The model under review builds one solid part; all positions refer to its coordinate system, in mm. Face numbers are marked on the shaded views. Coordinates: 2 decimals unless noted, no trailing zeros. Loops run counter-clockwise (first coordinate to the right, second up) from the corner with the lowest first, then second, coordinate; pieces in that order, holes last. Notation, with made-up numbers: M -32.75,39.25 L -19.75,39.25 A12 cw -19.75,43.25 Z; hole C -24.5,31.25 d10. An arc over 180 degrees is marked long. Return JSON: item names as keys, results as strings.
Autodesk Inventor part; units mm, degrees
ref_plane "YZ Plane" through (0, 0, 0) normal (1, 0, 0) x (0, 1, 0)
ref_plane "XZ Plane" through (0, 0, 0) normal (0, 1, 0) x (-1, 0, 0)
ref_plane "XY Plane" through (0, 0, 0) normal (0, 0, 1) x (1, 0, 0)
sketch "Sketch1" plane through (0, 0, 0) normal (0, 1, 0) x (-1, 0, 0)
  line L0 (0, 0) -> (0, -55.5) construction
  circle A0 centre (0, -55.5) radius 8
  line L1 (0, 0) -> (10, 0) construction
  line L2 (0, 0) -> (-10, 0) construction
  line L3 (10, -55.5) -> (10, 0)
  line L4 (-10, -55.5) -> (-10, 0)
  line L5 (0, 0) -> (0, -12.5) construction
  line L6 (0, -12.5) -> (0, -37.5) construction
  line L7 (0, -65.5) -> (0, -69.5) construction
  line L8 (0, -69.5) -> (3.25, -69.5)
  line L9 (4, -68.75) -> (4, -67.5)
  line L10 (0, -69.5) -> (-3.25, -69.5)
  line L11 (-4, -68.75) -> (-4, -67.5)
  arc A1 (-10, -55.5) -> (-6, -63.5) centre (0, -55.5) ccw
  arc A2 (6, -63.5) -> (10, -55.5) centre (0, -55.5) ccw
  arc A3 (6, -63.5) -> (4, -67.5) centre (9, -67.5) ccw
  arc A4 (-4, -67.5) -> (-6, -63.5) centre (-9, -67.5) ccw
  arc A5 (-4, -68.75) -> (-3.25, -69.5) centre (-3.25, -68.75) ccw
  arc A6 (3.25, -69.5) -> (4, -68.75) centre (3.25, -68.75) ccw
  line L12 (0, 0) -> (0, 55.5) construction
  circle A7 centre (0, 55.5) radius 8
  line L13 (10, 55.5) -> (10, 0)
  line L14 (-10, 55.5) -> (-10, 0)
  line L15 (0, 0) -> (0, 12.5) construction
  line L16 (0, 12.5) -> (0, 37.5) construction
  line L17 (0, 65.5) -> (0, 69.5) construction
  line L18 (0, 69.5) -> (3.25, 69.5)
  line L19 (4, 68.75) -> (4, 67.5)
  line L20 (0, 69.5) -> (-3.25, 69.5)
  line L21 (-4, 68.75) -> (-4, 67.5)
  arc A8 (-6, 63.5) -> (-10, 55.5) centre (0, 55.5) ccw
  arc A9 (10, 55.5) -> (6, 63.5) centre (0, 55.5) ccw
  arc A10 (4, 67.5) -> (6, 63.5) centre (9, 67.5) ccw
  arc A11 (-6, 63.5) -> (-4, 67.5) centre (-9, 67.5) ccw
  arc A12 (-3.25, 69.5) -> (-4, 68.75) centre (-3.25, 68.75) ccw
  arc A13 (4, 68.75) -> (3.25, 69.5) centre (3.25, 68.75) ccw
  point P0 (4, -69.5)
  point P1 (4, -64.6652)
  point P2 (-4, -69.5)
  point P3 (-4, -64.6652)
  point P4 (4, 69.5)
  point P5 (4, 64.6652)
  point P6 (-4, 69.5)
  point P7 (-4, 64.6652)
  dimension "d0" = 55.5
  dimension "d1" = 16
  dimension "d3" = 10
  dimension "d4" = 10
  dimension "d6" = 12.5
  dimension "d7" = 25
  dimension "d10" = 4
  dimension "d11" = 4
  dimension "d12" = 4
  dimension "d13" = 5
  dimension "d14" = 0.75
extrude "Extrusion1" add sketch "Sketch1" along normal blind 25
sketch "Sketch2" plane through (0, 0, 0) normal (0, 0, 1) x (1, 0, 0)
  line L0 (-10, 25) -> (10, 18.5016)
  line L1 (10, 0) -> (10, 25)
  line L2 (-10, 25) -> (11.0292, 25) construction
  line L3 (10, 18.5016) -> (10, 25)
  line L4 (10, 25) -> (-10, 25)
  point P0 (0, 0)
  dimension "d17" = 18
extrude "Extrusion2" cut sketch "Sketch2" along normal through all both and the other way through all
sketch "Sketch3" plane through (10, 18.5016, 55.5) normal (0.309, 0.9511, 0) x (0.9511, -0.309, 0)
  ellipse E0 centre (-10.5146, 0) end of major axis (-2.1029, 0) minor radius 8
  ellipse E1 centre (-10.5146, 111) end of major axis (-2.1029, 111) minor radius 8
  line L0 (-10.5146, 0) -> (-10.5146, 111) construction
  line L1 (-10.5146, 55.5) -> (-10.5146, 43)
  line L2 (-10.5146, 43) -> (-10.5146, 18)
  line L3 (-10.5146, 55.5) -> (-10.5146, 68)
  line L4 (-10.5146, 68) -> (-10.5146, 93)
  circle A0 centre (-10.5146, 18) radius 2
  circle A1 centre (-10.5146, 43) radius 2
  circle A2 centre (-10.5146, 68) radius 2
  circle A3 centre (-10.5146, 93) radius 2
  point P0 (-3.7933, 55.5)
  dimension "d20" = 12.5
  dimension "d21" = 25
  dimension "d22" = 12.5
  dimension "d23" = 25
  dimension "d24" = 4
  dimension "d25" = 4
  dimension "d26" = 4
  dimension "d27" = 4
extrude "Extrusion3" cut sketch "Sketch3" against normal blind 10 contours A0 | A1 L2 L1 | L1 L2 A1 | A3 | A2 L4 L3 | L3 L4 A2
sketch "Sketch4" plane through (10, 18.5016, 55.5) normal (0.309, 0.9511, 0) x (0.9511, -0.309, 0)
  circle A0 centre (-10.5146, 18) radius 2
  circle A1 centre (-10.5146, 18) radius 3
  circle A2 centre (-10.5146, 43) radius 2
  circle A3 centre (-10.5146, 43) radius 3
  circle A4 centre (-10.5146, 68) radius 2
  circle A5 centre (-10.5146, 68) radius 3
  circle A6 centre (-10.5146, 93) radius 2
  circle A7 centre (-10.5146, 93) radius 3
  point P0 (-3.7933, 55.5)
  dimension "d30" = 6
  dimension "d31" = 6
  dimension "d32" = 6
  dimension "d33" = 6
extrude "Extrusion4" cut sketch "Sketch4" against normal blind 1
sketch "Sketch5" plane through (-3.25, 0, 69.5) normal (0, 0, 1) x (1, 0, 0)
  line L0 (3.25, 0) -> (3.25, 5)
  line L1 (3.25, 5) -> (3.25, 15)
  circle A0 centre (3.25, 15) radius 1.75
  circle A1 centre (3.25, 5) radius 1.75
  dimension "d36" = 5
  dimension "d37" = 10
  dimension "d38" = 3.5
  dimension "d39" = 3.5
extrude "Extrusion5" cut sketch "Sketch5" against normal blind 7.5
sketch "Sketch6" plane through (3.25, 0, -69.5) normal (0, 0, -1) x (-1, 0, 0)
  line L0 (3.25, 0) -> (3.25, 5)
  line L1 (3.25, 5) -> (3.25, 15)
  circle A0 centre (3.25, 15) radius 1.75
  circle A1 centre (3.25, 5) radius 1.75
  dimension "d42" = 5
  dimension "d43" = 10
  dimension "d44" = 3.5
  dimension "d45" = 3.5
extrude "Extrusion6" cut sketch "Sketch6" against normal blind 7.5
chamfer "Chamfer1" distance 0.25 angle 45 4 edges at (1.75, 5, -69.5) (1.75, 15, -69.5) (-1.75, 15, 69.5) (-1.75, 5, 69.5)
properties part number "Leg_Battery_Connector"
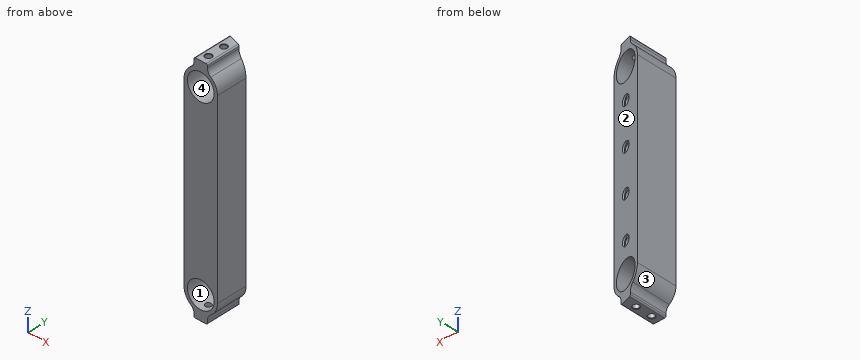
1. To check wall thickness, follow line 1 (Y direction, x = 0, z = 67.6); line 2 (Z direction, x = 3, y = 15.5); line 3 (Z direction, x = -5, y = 6) (3 decimals). State the ranges of each line that lie inside material, in increasing order.
Check values:
{"line 1": "0 to 3.25, 6.75 to 13.25, 16.75 to 21.75", "line 2": "-69.5 to -62.92, -48.08 to 48.08, 62.92 to 69.5", "line 3": "-64.5 to -61.745, -49.255 to 49.255, 61.745 to 64.5"}
2. Add section B-B on z = 57.5. Give the boundary of the cut face in (x, y), plus the area to 3 significant figures.
Check values:
{"outline": "M -9.8,0 L -7.75,0 L -7.75,24.27 L -9.8,24.93 Z; M 7.75,0 L 9.8,0 L 9.8,18.57 L 7.75,19.23 Z", "area": "89.3 mm²"}
3. The part is to be moulded in two halves that separate along Z. For the marked faces 1, 2, 3 and 4, say which applies: released by +Z, released by -Z, zero draft, split by the parting line, or undercut.
Check values:
{"face 1": "undercut", "face 2": "zero draft", "face 3": "released by -Z", "face 4": "undercut"}
4. Add section D-D on z = 23. Give the boundary of the cut face in (x, y).
Check values:
{"outline": "M -10,0 L 10,0 L 10,18.5 L -10,25 Z"}
5. Add section A-A on y = 9.75. Give the boundary of the cut face in (x, z), plus the area to 3 significant figures.
Check values:
{"outline": "M -10,-55.5 A10 ccw -6,-63.5 A5 cw -4,-67.5 L -4,-68.75 A0.75 ccw -3.25,-69.5 L 3.25,-69.5 A0.75 ccw 4,-68.75 L 4,-67.5 A5 cw 6,-63.5 A10 ccw 10,-55.5 L 10,55.5 A10 ccw 6,63.5 A5 cw 4,67.5 L 4,68.75 A0.75 ccw 3.25,69.5 L -3.25,69.5 A0.75 ccw -4,68.75 L -4,67.5 A5 cw -6,63.5 A10 ccw -10,55.5 Z; hole C 0,-55.5 d16; hole C 0,55.5 d16", "area": "2,200 mm²"}
6. Insertion check: pin 1 Ø0.6 at (y, z) = (15.5, -68) entering from -X; pin 2 Ø8 at (x, z) = (5.5, 14) entering from +Y; pin 3 Ø2 at (x, y) = (0, 15) entering from +Z; pin 4 Ø9.5 at (x, z) = (0, 55.5) entering from -Y. Each pin has a flat end and moves straight along its axis. Give the tip position at first contact, or say it passes through.
Check values:
{"pin 1": "x = -4", "pin 2": "y = 21.22", "pin 3": "z = 47.56", "pin 4": "through"}
7. Add section C-C on x = 0. State how many separate pieces and enclosed holes the cut face has, plus the area to 3 significant figures.
Check values:
{"separate pieces": "7", "enclosed holes": "0", "area": "2,150 mm²"}
